Could you check a few things on this model? Use its own coordinates, in mm. Face numbers are marked on the shaded views. A direction names the side the tool comes from. Give positions to 0.01 mm unless a question says otherwise; leave off trailing zeros. Order: outer loops, then holes, each group sorted by start corner. A loop starts at its lowest first (then second) coordinate and runs counter-clockwise, first axis right, second up.
(1) Will these pins go through, and if not, where does the flat tip stop? pin 1 (5.5 mm diameter, centred on x = 1.5, z = 41.5, fed in from -Y); pin 2 (1.5 mm diameter, centred on y = -1.5, z = 43, fed in from -X); pin 3 (5 mm diameter, centred on x = 0.5, y = -2.5, fed in from -Z).
(2) If we mould it in two halves opening along Y, with no side actions, what happens to the marked faces 5, 6 and 7? For each: released by +Y, released by -Y, zero draft, split by the parting line, or undercut.
(3) Imagine slicing it at D-D, the plane y = 5. Write out the boundary of the cut face in (x, z).
(4) Imagine slicing it at B-B, the plane y = -1. Write out the boundary of the cut face in (x, z).
(5) If I drill on probe 1 along Y at (x, z) = (-6, 9); probe 2 along Z at (x, y) = (0, 2.5), over which ranges is the centre line in solid material (lowest first)?
(6) Imagine slicing it at A-A, the plane z = 5. Write out the boundary of the cut face in (x, y), then the cut area to 3 significant figures.
(7) On a 3-axis mill with a long thin cutter (end or side, diameter ignored), from which of +Z, -Z, +X, -X, +Y, -Y can I reach the whole of each face in a straight line? I mean the marked faces 1, 2, 3 and 4. Say none if no direction works.
from build123d import *

# Parameters (mm, degrees)
SKETCH_W     = 15
SKETCH_H     = 15
PAD_DEPTH    = 40
SKETCH001_W  = 12.1
SKETCH001_H  = 12.1
POCKET_DEPTH = 30
SKETCH002_W  = 7.8
SKETCH002_H  = 7.8
PAD001_DEPTH = 5
CHAMFER_SIZE = 3


with BuildPart() as part:
    # Sketch → Pad (new body)
    with BuildSketch(Plane.XY):
        Rectangle(SKETCH_W, SKETCH_H)
    extrude(amount=PAD_DEPTH)

    # Sketch001 (on Face5 of Pad) → Pocket (cut)
    with BuildSketch(Plane(origin=(0, 0, 0), x_dir=(1, 0, 0), z_dir=(0, 0, -1))):
        Rectangle(SKETCH001_W, SKETCH001_H)
    extrude(amount=-POCKET_DEPTH, mode=Mode.SUBTRACT)

    # Sketch002 (on Face5 of Pocket) → Pad001 (join)
    with BuildSketch(Plane.XY.offset(40)):
        Rectangle(SKETCH002_W, SKETCH002_H)
    extrude(amount=PAD001_DEPTH)

    # Chamfer
    chamfer_edges = [part.edges().sort_by_distance(p)[0] for p in [
        (-7.5, 0, 40),
        (0, 7.5, 40),
        (7.5, 0, 40),
        (0, -7.5, 40),
    ]]
    chamfer(chamfer_edges, length=CHAMFER_SIZE)


solid = part.part
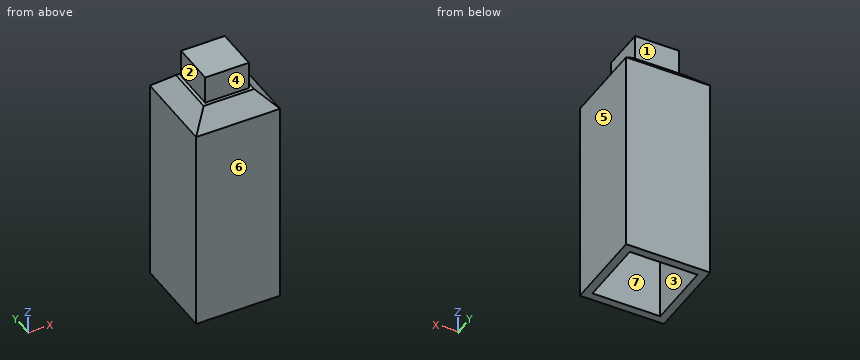
Answer block:
1. pin 1: stops at y = -5.75
1. pin 2: stops at x = -3.9
1. pin 3: stops at z = 30
2. face 5: zero draft
2. face 6: released by -Y
2. face 7: undercut
3. outline: (-7.5, 0) - (-6.05, 0) - (-6.05, 30) - (6.05, 30) - (6.05, 0) - (7.5, 0) - (7.5, 37) - (5, 39.5) - (-5, 39.5) - (-7.5, 37) - close
4. outline: (-7.5, 0) - (-6.05, 0) - (-6.05, 30) - (6.05, 30) - (6.05, 0) - (7.5, 0) - (7.5, 37) - (4.5, 40) - (3.9, 40) - (3.9, 45) - (-3.9, 45) - (-3.9, 40) - (-4.5, 40) - (-7.5, 37) - close
5. probe 1: y = -7.5 to -6.05, 6.05 to 7.5
5. probe 2: z = 30 to 45
6. outline: (-7.5, -7.5) - (7.5, -7.5) - (7.5, 7.5) - (-7.5, 7.5) - close; hole (-6.05, -6.05) - (6.05, -6.05) - (6.05, 6.05) - (-6.05, 6.05) - close
6. area: 78.6 mm2
7. face 1: +Z, +X, -X, +Y
7. face 2: +Z, -X, +Y, -Y
7. face 3: -Z
7. face 4: +Z, +X, -X, -Y
